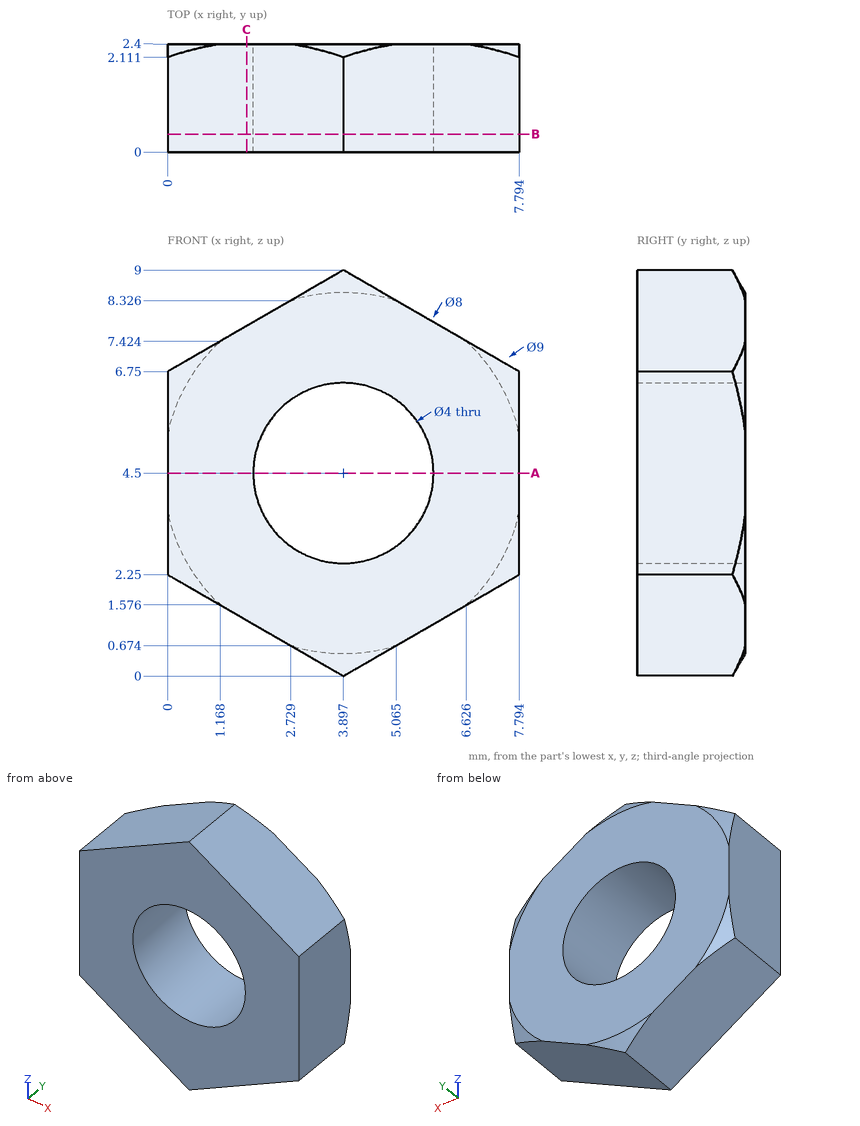
Design review of the part shown in the three views and the two pictorial views. Dimensions are in mm from the part's minimum x, y and z. Round coordinates to 2 decimals unless told otherwise and drop trailing zeros. Order: outer loops, then holes, each group sorted by start corner. A loop starts at its lowest first (then second) coordinate and runs counter-clockwise, first axis right, second up.
(1) Take a section at C-C, the plane x = 1.75. State the section outline as (y, z) points.
Working result:
outline: (0, 1.24) - (2.4, 1.24) - (2.4, 7.76) - (0, 7.76) - close
(2) Take a section at A-A, the plane z = 4.5. State the section outline as (x, y) points.
Working result:
outline: (0, 0) - (1.9, 0) - (1.9, 2.4) - (0, 2.4) - close; (5.9, 0) - (7.79, 0) - (7.79, 2.4) - (5.9, 2.4) - close
(3) Take a section at B-B, the plane y = 0.4. State the section outline as (x, z) points.
Working result:
outline: (0, 2.25) - (3.9, 0) - (7.79, 2.25) - (7.79, 6.75) - (3.9, 9) - (0, 6.75) - close; hole circle Ø4 at (3.9, 4.5)
(4) Wall thickness on L1, parallel to X at y = 1.95, z = 2.75 (1 decimal); L2, parallel to X at y = 1.55, z = 3.5 (1 decimal); L3, parallel to Z at x = 5, y = 0.1: over which ranges is each line inside the solid? List them lowest first.
Working result:
L1: x = 0 to 2.9, 4.9 to 7.8
L2: x = 0 to 2.2, 5.6 to 7.8
L3: z = 0.64 to 2.83, 6.17 to 8.36
(5) For P1, Ø3, axis at x = 3.9, z = 4.5, coming from the +Y side, flat-tipped, find the tip position at first contact; note if it passes through.
Working result:
P1: passes through
